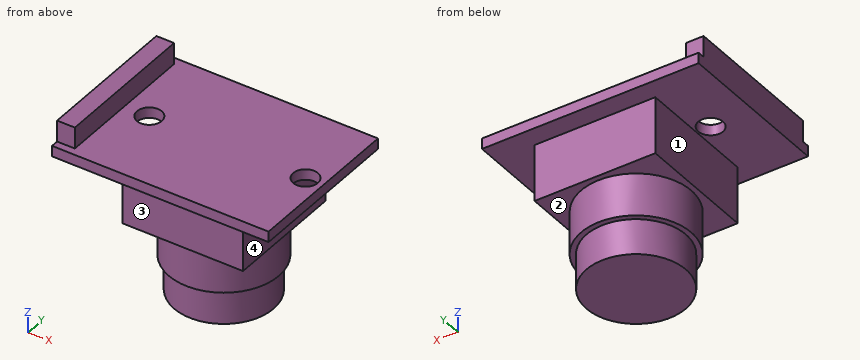
from build123d import *

# Parameters (mm, degrees)
SKETCH_1_R      = 7
EXTRUDE_1_DEPTH = 5
SKETCH_2_R      = 7.75
EXTRUDE_2_DEPTH = 6
SKETCH_3_W      = 17
SKETCH_3_H      = 17
EXTRUDE_3_DEPTH = 8
SKETCH_4_W      = 30.5
SKETCH_4_H      = 22.6
SKETCH_4_R      = 1.75
EXTRUDE_4_DEPTH = 1.5
SKETCH_5_W      = 2.5
SKETCH_5_H      = 20.5
EXTRUDE_5_DEPTH = 3


with BuildPart() as part:
    # 草图1 → 凸台-拉伸1 (new body)
    with BuildSketch(Plane.XY):
        Circle(SKETCH_1_R)
    extrude(amount=EXTRUDE_1_DEPTH)

    # 草图2 → 凸台-拉伸2 (add)
    with BuildSketch(Plane.XY.offset(5)):
        Circle(SKETCH_2_R)
    extrude(amount=EXTRUDE_2_DEPTH)

    # 草图3 → 凸台-拉伸3 (add)
    with BuildSketch(Plane.XY.offset(11)):
        Rectangle(SKETCH_3_W, SKETCH_3_H)
    extrude(amount=EXTRUDE_3_DEPTH)

    # 草图4 → 凸台-拉伸4 (add)
    with BuildSketch(Plane.XY.offset(19)):
        with Locations((-1.25, 0)):
            Rectangle(SKETCH_4_W, SKETCH_4_H)
        with Locations((11.5, 0)):
            Circle(SKETCH_4_R, mode=Mode.SUBTRACT)
        with Locations((-10.5, 0)):
            Circle(SKETCH_4_R, mode=Mode.SUBTRACT)
    extrude(amount=EXTRUDE_4_DEPTH)

    # 草图5 → 凸台-拉伸5 (add)
    with BuildSketch(Plane.XY.offset(20.5)):
        with Locations((-15.25, 0)):
            Rectangle(SKETCH_5_W, SKETCH_5_H)
    extrude(amount=EXTRUDE_5_DEPTH)


solid = part.part
For this review, take the finished solid that the model builds, in its own axes (mm). Face numbers are marked on the shaded views. A direction names the side the tool comes from. Give positions to 0.01 mm unless a question says otherwise; leave off trailing zeros. Loops run counter-clockwise (first coordinate to the right, second up) from the corner with the lowest first, then second, coordinate; pieces in that order, holes last. Notation, with made-up numbers: (66.5, 71) - (77.5, 71) arc R22 cw to (77.5, 86) - close; hole circle Ø8 at (79.5, 48.25). An arc over 180 degrees is marked (long way). Write each question's results on one line, items separated by ' | '.
(1) Take a section at B-B (y = 0). Give the boundary of the cut face in (x, z).
Conclusion:
outline: (-16.5, 19) - (-12.25, 19) - (-12.25, 20.5) - (-14, 20.5) - (-14, 23.5) - (-16.5, 23.5) - close; (-8.75, 19) - (-8.5, 19) - (-8.5, 11) - (-7.75, 11) - (-7.75, 5) - (-7, 5) - (-7, 0) - (7, 0) - (7, 5) - (7.75, 5) - (7.75, 11) - (8.5, 11) - (8.5, 19) - (9.75, 19) - (9.75, 20.5) - (-8.75, 20.5) - close; (13.25, 19) - (14, 19) - (14, 20.5) - (13.25, 20.5) - close
(2) Take a section at D-D (y = -9.25). Give the boundary of the cut face in (x, z), then the cut area to 4 significant figures.
Conclusion:
outline: (-16.5, 19) - (14, 19) - (14, 20.5) - (-14, 20.5) - (-14, 23.5) - (-16.5, 23.5) - close | area: 53.25 mm^2
(3) For the marked faces 1, 2, 3 and 4, list the 3-axis set-ups (+Z, -Z, +X, -X, +Y, -Y) from which the entire face can be reached by the end or side of a thin tool; tool diameter is ignored.
Conclusion:
face 1: -Z, -X, +Y, -Y | face 2: -Z | face 3: -Z, +X, -X, -Y | face 4: -Z, +X, +Y, -Y
(4) Take a section at C-C (x = 0). Give the boundary of the cut face in (y, z), then the cut area to 3 significant figures.
Conclusion:
outline: (-11.3, 19) - (-8.5, 19) - (-8.5, 11) - (-7.75, 11) - (-7.75, 5) - (-7, 5) - (-7, 0) - (7, 0) - (7, 5) - (7.75, 5) - (7.75, 11) - (8.5, 11) - (8.5, 19) - (11.3, 19) - (11.3, 20.5) - (-11.3, 20.5) - close | area: 333 mm^2
(5) Take a section at A-A (x = 11.5). Give the boundary of the cut face in (y, z).
Conclusion:
outline: (-11.3, 19) - (-1.75, 19) - (-1.75, 20.5) - (-11.3, 20.5) - close; (1.75, 19) - (11.3, 19) - (11.3, 20.5) - (1.75, 20.5) - close
(6) For pin 1 Ø4 at (x, z) = (8, 15.5) entering from +Y; pin 2 Ø0.8 at (x, z) = (-14.5, 22) entering from -Y; pin 3 Ø2 at (x, z) = (-15.5, 22) entering from +Y, all flat-tipped, find the tip position at first contact; note any pin that passes through.
Conclusion:
pin 1: y = 8.5 | pin 2: y = -10.25 | pin 3: y = 10.25
(7) For line 1 along Y through (x, z) = (-10.5, 20); line 2 along X through (y, z) = (-0.25, 19.5); line 3 along Z through (x, y) = (8, 6.25), list the stretches that pass through material, from the lowest coordinate up.
Conclusion:
line 1: -11.3 to -1.75, 1.75 to 11.3 | line 2: -16.5 to -12.23, -8.77 to 9.77, 13.23 to 14 | line 3: 11 to 20.5
